Source: CAD feature listing. Evaluate the final solid. Frame: model axes, mm. Face numbers are marked on the shaded views. Round coordinates to 2 decimals unless told otherwise and drop trailing zeros. Order: outer loops, then holes, each group sorted by start corner. A loop starts at its lowest first (then second) coordinate and runs counter-clockwise, first axis right, second up. Notation, with made-up numbers: (41, 20.5) -> (77, 20.5) arc R13 cw to (77, 39.5) -> close; hole circle Ø1 at (87.25, 31.25). An arc over 180 degrees is marked (long way). One line per item, written item: value. Start each with the question number.
1) Section C-C (y = -30). Return the cut outline in (x, z), and give its area (3 significant figures).
2) Section B-B (z = 4). Return the cut outline in (x, y), and give its area (3 significant figures).
3) Ray query, L1, parallel to Y at x = 9.5, z = 15; L2, parallel to Y at x = -19.5, z = 19; L3, parallel to X at y = -49, z = 21.5. Return the intervals inside material, ascending.
4) Section D-D (x = 13). Return the cut outline in (y, z), and give its area (3 significant figures).
5) Section A-A (x = -20). Return the cut outline in (y, z), and give its area (3 significant figures).
6) Mould query, pull axis Z, two halves, no side actions, for the marked faces 1, 2 and 3. Classes: pulls with the +Z half, pulls with the -Z half, needs draft (parallel to the pull), parting line crosses it, or undercut.
7) Pin query (flat end, axial travel): P1, Ø3, axis at x = -31.5, y = -47.5, coming from the -Z side; P2, Ø3.5, axis at x = -20, y = 15, coming from the +Z side; P3, Ø3, axis at x = 34.5, y = 47.5, coming from the -Z side; P4, Ø3, axis at y = 16, z = 19.5, coming from the +X side. Return the tip coordinate at first contact, or that it passes through.
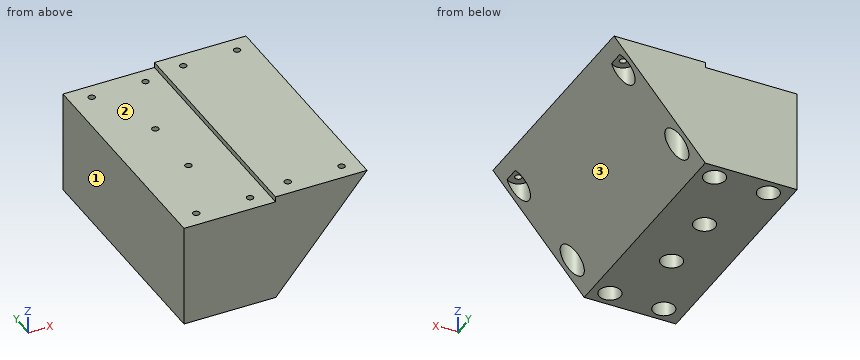
```python
from build123d import *

# Parameters (mm, degrees)
SKETCH1_W           = 85
SKETCH1_H           = 110
BOSS_EXTRUDE1_DEPTH = 50.5
SKETCH2_W           = 42.5
SKETCH2_H           = 110
CUT_EXTRUDE1_DEPTH  = 2.5
CUT_EXTRUDE2_REACH  = 87.988
SKETCH3_W           = 130
SKETCH3_H           = 130
CUT_EXTRUDE3_REACH  = 86.47
SKETCH4_R           = 1.55
SKETCH5_R           = 1.55
CUT_EXTRUDE5_DEPTH  = 86.915656315
SKETCH9_R           = 5
CUT_EXTRUDE6_DEPTH  = 55
SKETCH10_R          = 5
CUT_EXTRUDE7_DEPTH  = 40


with BuildPart() as part:
    # Sketch1 → Boss-Extrude1 (new body)
    with BuildSketch(Plane.XY):
        Rectangle(SKETCH1_W, SKETCH1_H)
    extrude(amount=BOSS_EXTRUDE1_DEPTH)

    # Sketch2 → Cut-Extrude1 (cut)
    with BuildSketch(Plane.XY.offset(50.5)):
        with Locations((-21.25, 0)):
            Rectangle(SKETCH2_W, SKETCH2_H)
    extrude(amount=-CUT_EXTRUDE1_DEPTH, mode=Mode.SUBTRACT)

    # Sketch3 → Cut-Extrude2 (cut, up to next)
    with BuildSketch(Plane(origin=(0.073628012, 0, -0.061781238), x_dir=(0, 1, 0), z_dir=(-0.7660444431189792, 0, 0.6427876096865379)), mode=Mode.PRIVATE) as cut_extrude2_sk1:
        with Locations((-1.816321809, -4.4988995)):
            Rectangle(SKETCH3_W, SKETCH3_H)
    cut_extrude2_tool1 = extrude(cut_extrude2_sk1.sketch, amount=-CUT_EXTRUDE2_REACH, mode=Mode.PRIVATE) & part.part
    add(cut_extrude2_tool1.solids().sort_by_distance((2.965465, -1.816322, 3.384576))[0], mode=Mode.SUBTRACT)

    # Sketch4 → Cut-Extrude3 (cut, up to next)
    with BuildSketch(Plane.XY.offset(48), mode=Mode.PRIVATE) as cut_extrude3_sk1:
        with Locations((-8, 47.5)):
            Circle(SKETCH4_R)
    cut_extrude3_tool1 = extrude(cut_extrude3_sk1.sketch, amount=-CUT_EXTRUDE3_REACH, mode=Mode.PRIVATE) & part.part
    # Sketch4 → Cut-Extrude3 (cut, up to next)
    with BuildSketch(Plane.XY.offset(48), mode=Mode.PRIVATE) as cut_extrude3_sk2:
        with Locations((-33, 47.5)):
            Circle(SKETCH4_R)
    cut_extrude3_tool2 = extrude(cut_extrude3_sk2.sketch, amount=-CUT_EXTRUDE3_REACH, mode=Mode.PRIVATE) & part.part
    # Sketch4 → Cut-Extrude3 (cut, up to next)
    with BuildSketch(Plane.XY.offset(48), mode=Mode.PRIVATE) as cut_extrude3_sk3:
        with Locations((-20, 15)):
            Circle(SKETCH4_R)
    cut_extrude3_tool3 = extrude(cut_extrude3_sk3.sketch, amount=-CUT_EXTRUDE3_REACH, mode=Mode.PRIVATE) & part.part
    # Sketch4 → Cut-Extrude3 (cut, up to next)
    with BuildSketch(Plane.XY.offset(48), mode=Mode.PRIVATE) as cut_extrude3_sk4:
        with Locations((-20, -15)):
            Circle(SKETCH4_R)
    cut_extrude3_tool4 = extrude(cut_extrude3_sk4.sketch, amount=-CUT_EXTRUDE3_REACH, mode=Mode.PRIVATE) & part.part
    # Sketch4 → Cut-Extrude3 (cut, up to next)
    with BuildSketch(Plane.XY.offset(48), mode=Mode.PRIVATE) as cut_extrude3_sk5:
        with Locations((-8, -47.5)):
            Circle(SKETCH4_R)
    cut_extrude3_tool5 = extrude(cut_extrude3_sk5.sketch, amount=-CUT_EXTRUDE3_REACH, mode=Mode.PRIVATE) & part.part
    # Sketch4 → Cut-Extrude3 (cut, up to next)
    with BuildSketch(Plane.XY.offset(48), mode=Mode.PRIVATE) as cut_extrude3_sk6:
        with Locations((-33, -47.5)):
            Circle(SKETCH4_R)
    cut_extrude3_tool6 = extrude(cut_extrude3_sk6.sketch, amount=-CUT_EXTRUDE3_REACH, mode=Mode.PRIVATE) & part.part
    add(cut_extrude3_tool1.solids().sort_by_distance((-8, 47.5, 48))[0], mode=Mode.SUBTRACT)
    add(cut_extrude3_tool2.solids().sort_by_distance((-33, 47.5, 48))[0], mode=Mode.SUBTRACT)
    add(cut_extrude3_tool3.solids().sort_by_distance((-20, 15, 48))[0], mode=Mode.SUBTRACT)
    add(cut_extrude3_tool4.solids().sort_by_distance((-20, -15, 48))[0], mode=Mode.SUBTRACT)
    add(cut_extrude3_tool5.solids().sort_by_distance((-8, -47.5, 48))[0], mode=Mode.SUBTRACT)
    add(cut_extrude3_tool6.solids().sort_by_distance((-33, -47.5, 48))[0], mode=Mode.SUBTRACT)

    # Sketch5 → Cut-Extrude5 (cut, through all)
    with BuildSketch(Plane.XY.offset(50.5)):
        with Locations((9.5, 47.5)):
            Circle(SKETCH5_R)
        with Locations((34.5, 47.5)):
            Circle(SKETCH5_R)
        with Locations((34.5, -47.5)):
            Circle(SKETCH5_R)
        with Locations((9.5, -47.5)):
            Circle(SKETCH5_R)
    extrude(amount=-CUT_EXTRUDE5_DEPTH, mode=Mode.SUBTRACT)

    # Sketch9 → Cut-Extrude6 (cut)
    with BuildSketch(Plane(origin=(0, 0, -10), x_dir=(-1, 0, 0), z_dir=(0, 0, -1))):
        with Locations((-34.5, 47.5)):
            Circle(SKETCH9_R)
        with Locations((-9.5, 47.5)):
            Circle(SKETCH9_R)
        with Locations((-34.5, -47.5)):
            Circle(SKETCH9_R)
        with Locations((-9.5, -47.5)):
            Circle(SKETCH9_R)
    extrude(amount=-CUT_EXTRUDE6_DEPTH, mode=Mode.SUBTRACT)

    # Sketch10 → Cut-Extrude7 (cut)
    with BuildSketch(Plane(origin=(0, 0, 0), x_dir=(-1, 0, 0), z_dir=(0, 0, -1))):
        with Locations((8, 47.5)):
            Circle(SKETCH10_R)
        with Locations((33, 47.5)):
            Circle(SKETCH10_R)
        with Locations((33, -47.5)):
            Circle(SKETCH10_R)
        with Locations((8, -47.5)):
            Circle(SKETCH10_R)
        with Locations((20, 15)):
            Circle(SKETCH10_R)
        with Locations((20, -15)):
            Circle(SKETCH10_R)
    extrude(amount=-CUT_EXTRUDE7_DEPTH, mode=Mode.SUBTRACT)


solid = part.part
```
Findings:
1. outline: (-42.5, 0) -> (0.13, 0) -> (42.5, 50.5) -> (0, 50.5) -> (0, 48) -> (-42.5, 48) -> close
1. area: 3,120 mm2
2. outline: (-42.5, -55) -> (3.48, -55) -> (3.48, 55) -> (-42.5, 55) -> close; hole circle Ø10 at (-33, -47.5); hole circle Ø10 at (-33, 47.5); hole circle Ø10 at (-20, -15); hole circle Ø10 at (-20, 15); hole circle Ø10 at (-8, -47.5); hole circle Ø10 at (-8, 47.5)
2. area: 4,590 mm2
3. L1: -55 to -52.5, -42.5 to 42.5, 52.5 to 55
3. L2: -55 to -19.97, -10.03 to 10.03, 19.97 to 55
3. L3: -42.5 to -37.77, -28.23 to -12.77, -3.23 to 4.73, 14.27 to 18.17
4. outline: (-55, 15.34) -> (-51.07, 15.34) -> (-51.07, 45) -> (-43.93, 45) -> (-43.93, 15.34) -> (43.93, 15.34) -> (43.93, 45) -> (51.07, 45) -> (51.07, 15.34) -> (55, 15.34) -> (55, 50.5) -> (-55, 50.5) -> close
4. area: 3,440 mm2
5. outline: (-55, 0) -> (-20, 0) -> (-20, 40) -> (-16.55, 40) -> (-16.55, 48) -> (-55, 48) -> close; (-13.45, 40) -> (-10, 40) -> (-10, 0) -> (10, 0) -> (10, 40) -> (13.45, 40) -> (13.45, 48) -> (-13.45, 48) -> close; (16.55, 40) -> (20, 40) -> (20, 0) -> (55, 0) -> (55, 48) -> (16.55, 48) -> close
5. area: 4,430 mm2
6. face 1: needs draft
6. face 2: pulls with the +Z half
6. face 3: pulls with the -Z half
7. P1: z = 40
7. P2: z = 48
7. P3: through
7. P4: x = 17.75
